Design review of the part built by this model. Coordinates are the model's own, in mm. Face numbers are marked on the shaded views. Give positions to 0.01 mm unless a question says otherwise; leave off trailing zeros. Write each loop counter-clockwise with the first axis right and the second up, starting at its lowest first coordinate (ties: lowest second). Pieces come first, ordered by that corner, then holes. Notation, with made-up numbers: (-35, 68) -> (18, 68) arc R14 cw to (18, 84) -> close; hole circle Ø10 at (33.5, -18). An arc over 180 degrees is marked (long way). Use CSV: the item, a comma, the result in double quotes.
```python
from build123d import *

# Parameters (mm, degrees)
SKETCH1_W           = 22
SKETCH1_H           = 10
BOSS_EXTRUDE1_DEPTH = 9
FILLET2_R           = 0.5
CUT_EXTRUDE4_DEPTH  = 1
SKETCH8_W           = 2
SKETCH8_H           = 6.5
CUT_EXTRUDE5_DEPTH  = 1
CUT_EXTRUDE6_DEPTH  = 1
SKETCH14_R          = 0.45
SKETCH15_R          = 0.45
FILLET4_R           = 0.1


with BuildPart() as part:
    # Sketch1 → Boss-Extrude1 (new body)
    with BuildSketch(Plane.XY):
        with Locations((11, -5)):
            Rectangle(SKETCH1_W, SKETCH1_H)
    extrude(amount=BOSS_EXTRUDE1_DEPTH)

    # Fillet2
    fillet2_edges = [part.edges().sort_by_distance(p)[0] for p in [
        (11, 0, 9),
        (11, 0, 0),
        (11, -10, 0),
        (11, -10, 9),
    ]]
    fillet(fillet2_edges, radius=FILLET2_R)

    # 3DSketch1 → Cut-Extrude4 (cut)
    with BuildSketch(Plane(origin=(22, -10, 5.5), x_dir=(0, 0.9557790087219501, -0.29408584883752314), z_dir=(1, 0, 0))):
        Polygon((0, 0), (6.212563557, 1.911558017), (6.800735254, 0), (0.588171698, -1.911558017), align=None)
    extrude(amount=-CUT_EXTRUDE4_DEPTH, mode=Mode.SUBTRACT)

    # Sketch8 → Cut-Extrude5 (cut)
    with BuildSketch(Plane.ZY):
        with Locations((4.5, -6.75)):
            Rectangle(SKETCH8_W, SKETCH8_H)
    extrude(amount=-CUT_EXTRUDE5_DEPTH, mode=Mode.SUBTRACT)

    # Sketch6 → Cut-Extrude6 (cut)
    with BuildSketch(Plane.XZ.offset(10)):
        Polygon((1, 5.5), (1, 3.5), (3, 3.5), (3, 1), (19, 1), (19, 3.5), (21, 3.5), (21, 5.5), (19, 5.5), (19, 8), (3, 8), (3, 5.5), align=None)
    extrude(amount=-CUT_EXTRUDE6_DEPTH, mode=Mode.SUBTRACT)

    # Sweep2: sweep along a curve in space
    with BuildLine() as sweep2_path:
        Line((21, -5, 4.5), (23.5, -5, 4.5))
        ThreePointArc((24.5, -6, 4.5), (24.207106781, -5.292893219, 4.5), (23.5, -5, 4.5))
        Line((24.5, -6, 4.5), (24.5, -11, 4.5))
        ThreePointArc((23.5, -12, 4.5), (24.207106781, -11.707106781, 4.5), (24.5, -11, 4.5))
        Line((23.5, -12, 4.5), (-7.5, -12, 4.5))
    # Sketch14 → Sweep2 (sweep)
    with BuildSketch(Plane(origin=(21, 0, 0), x_dir=(0, 0, -1), z_dir=(1, 0, 0))):
        with Locations((-4.5, -5)):
            Circle(SKETCH14_R)
    sweep(path=sweep2_path.line)

    # Sweep3: sweep along a curve in space
    with BuildLine() as sweep3_path:
        Line((1, -5, 4.5), (-7.5, -5, 4.5))
    # Sketch15 → Sweep3 (sweep)
    with BuildSketch(Plane.ZY.offset(-1)):
        with Locations((4.5, -5)):
            Circle(SKETCH15_R)
    sweep(path=sweep3_path.line)

    # Fillet4
    fillet4_edges = [part.edges().sort_by_distance(p)[0] for p in [
        (-7.5, -12, 4.95),
        (-7.5, -5, 4.05),
    ]]
    fillet(fillet4_edges, radius=FILLET4_R)


solid = part.part
```
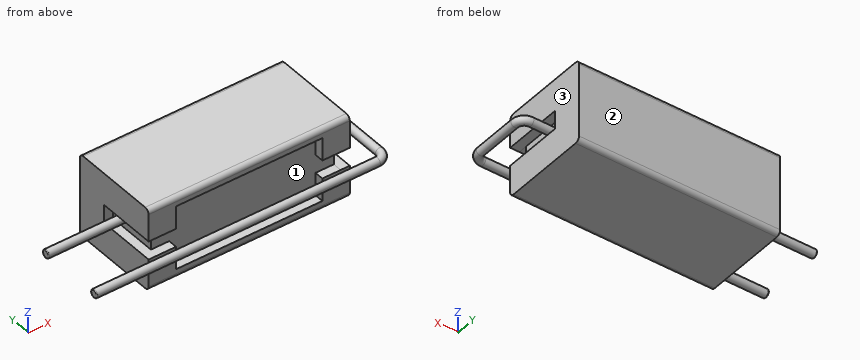
(1) Clearance check with flat-ended pins moving along their axes: pin 1 (0.9 mm diameter, centred on x = 13, z = 1.5, fed in from -Y); pin 2 (2 mm diameter, centred on y = -2, z = 2.5, fed in from +X). State where each tip first meets the part, or that it passes through.
Established:
pin 1,"stops at y = -9"
pin 2,"stops at x = 22"
(2) Mouldability with a two-part tool opening along X and no side actions: class the marked faces 1, 2 and 3 as +X half, -X half, draft (parallel to the pull), parting line (faces both ways), or undercut.
Established:
face 1,"undercut"
face 2,"draft"
face 3,"+X half"
(3) Take a section at A-A (x = 10). Write out the cut boundary in (y, z).
Established:
outline,"circle Ø0.9 at (-12, 4.5); (-10, 0.5) arc R0.5 ccw to (-9.5, 0) -> (-0.5, 0) arc R0.5 ccw to (0, 0.5) -> (0, 8.5) arc R0.5 ccw to (-0.5, 9) -> (-9.5, 9) arc R0.5 ccw to (-10, 8.5) -> (-10, 8) -> (-9, 8) -> (-9, 1) -> (-10, 1) -> close"
(4) Take a section at C-C (z = 4.5). Write out the cut boundary in (x, y).
Established:
outline,"(-7.5, -12.35) arc R0.1 ccw to (-7.4, -12.45) -> (23.5, -12.45) arc R1.45 ccw to (24.95, -11) -> (24.95, -6) arc R1.45 ccw to (23.5, -4.55) -> (21, -4.55) -> (21, -3.5) -> (22, -3.5) -> (22, 0) -> (0, 0) -> (0, -3.5) -> (1, -3.5) -> (1, -4.55) -> (-7.4, -4.55) arc R0.1 ccw to (-7.5, -4.65) -> (-7.5, -5.35) arc R0.1 ccw to (-7.4, -5.45) -> (1, -5.45) -> (1, -9) -> (21, -9) -> (21, -5.45) -> (23.5, -5.45) arc R0.55 cw to (24.05, -6) -> (24.05, -11) arc R0.55 cw to (23.5, -11.55) -> (-7.4, -11.55) arc R0.1 ccw to (-7.5, -11.65) -> close"
(5) For line 1 along Y through (x, z) = (20.5, 3); line 2 along X through (y, z) = (-7, 8); line 3 along Y through (x, z) = (5.5, 7.5), list the stretches that pass through material, from the lowest coordinate up. Write a range as [from, to].
Established:
line 1,"y = [-10, 0]"
line 2,"x = [0, 22]"
line 3,"y = [-9, 0]"
(6) Take a section at D-D (z = 6). Write out the cut boundary in (x, y).
Established:
outline,"(0, -10) -> (3, -10) -> (3, -9) -> (19, -9) -> (19, -10) -> (22, -10) -> (22, 0) -> (0, 0) -> close"
(7) Take a section at B-B (y = -8). Write out the cut boundary in (x, z).
Established:
outline,"(0, 0) -> (22, 0) -> (22, 3.5) -> (21, 3.5) -> (21, 5.5) -> (22, 5.5) -> (22, 9) -> (0, 9) -> (0, 5.5) -> (1, 5.5) -> (1, 3.5) -> (0, 3.5) -> close; circle Ø0.9 at (24.5, 4.5)"
